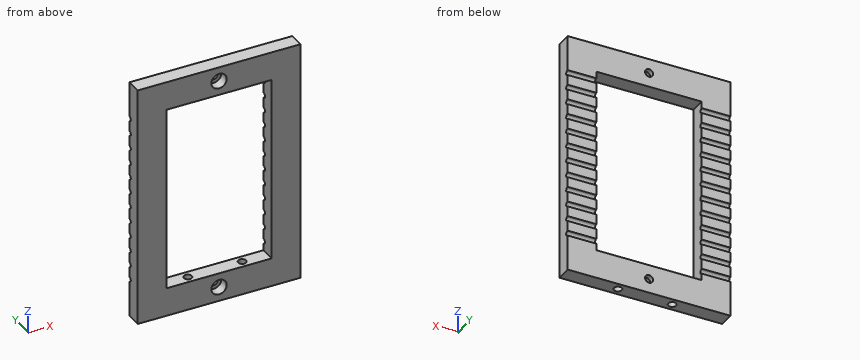
Autodesk Inventor part; units mm, degrees
ref_plane "YZ Plane" through (0, 0, 0) normal (1, 0, 0) x (0, 1, 0)
ref_plane "XZ Plane" through (0, 0, 0) normal (0, 1, 0) x (-1, 0, 0)
ref_plane "XY Plane" through (0, 0, 0) normal (0, 0, 1) x (1, 0, 0)
sketch "Sketch1" plane through (0, 0, 0) normal (0, 1, 0) x (-1, 0, 0)
  line L0 (0, 0) -> (101.6, 0)
  line L1 (101.6, 0) -> (101.6, -152.4)
  line L2 (101.6, -152.4) -> (0, -152.4)
  line L3 (0, -152.4) -> (0, 0)
  dimension "d0" = 101.6
  dimension "d1" = 152.4
extrude "Extrusion1" add sketch "Sketch1" along normal blind 9.525
sketch "Sketch2" plane through (0, 9.525, 0) normal (0, 1, 0) x (1, 0, 0)
  line L0 (-101.6, 0) -> (0, 0)
  line L1 (0, 0) -> (-17.9605, 17.9605)
  line L2 (0, 0) -> (25.4, 0) construction
  line L3 (-101.6, 152.4) -> (-101.6, 0)
  line L4 (-101.6, 152.4) -> (-83.6395, 134.4395)
  line L5 (-17.9605, 17.9605) -> (-83.6395, 17.9605)
  line L6 (-83.6395, 17.9605) -> (-83.6395, 134.4395)
  line L7 (-83.6395, 134.4395) -> (-17.9605, 134.4395)
  line L8 (-17.9605, 134.4395) -> (-17.9605, 17.9605)
  dimension "d4" = 25.4
  dimension "d5" = 135
  dimension "d6" = 25.4
extrude "Extrusion2" cut sketch "Sketch2" against normal blind 9.525 contours L5 L6 L7 L8
sketch "Sketch3" plane through (0, 0, 0) normal (1, 0, 0) x (0, 0, -1)
  line L0 (0, 9.525) -> (152.4, 9.525)
  line L1 (0, 10.079) -> (25.4, 10.079) construction
  line L2 (0, 0) -> (0, 9.525)
  line L3 (0, 9.525) -> (23.8125, 9.525)
  line L4 (134.4395, 9.525) -> (17.9605, 9.525)
  circle A0 centre (23.8125, 9.525) radius 1.5875
  circle A1 centre (33.3375, 9.525) radius 1.5875
  circle A2 centre (42.8625, 9.525) radius 1.5875
  circle A3 centre (52.3875, 9.525) radius 1.5875
  circle A4 centre (61.9125, 9.525) radius 1.5875
  circle A5 centre (71.4375, 9.525) radius 1.5875
  circle A6 centre (80.9625, 9.525) radius 1.5875
  circle A7 centre (90.4875, 9.525) radius 1.5875
  circle A8 centre (100.0125, 9.525) radius 1.5875
  circle A9 centre (109.5375, 9.525) radius 1.5875
  circle A10 centre (119.0625, 9.525) radius 1.5875
  circle A11 centre (128.5875, 9.525) radius 1.5875
  point P0 (130.175, 9.525)
  point P1 (127, 9.525)
  point P2 (120.65, 9.525)
  point P3 (117.475, 9.525)
  point P4 (101.6, 9.525)
  point P5 (98.425, 9.525)
  point P6 (82.55, 9.525)
  point P7 (79.375, 9.525)
  point P8 (73.025, 9.525)
  point P9 (69.85, 9.525)
  point P10 (63.5, 9.525)
  point P11 (60.325, 9.525)
  point P12 (53.975, 9.525)
  point P13 (50.8, 9.525)
  point P14 (44.45, 9.525)
  point P15 (41.275, 9.525)
  point P16 (34.925, 9.525)
  point P17 (31.75, 9.525)
  point P18 (22.225, 9.525)
  point P19 (25.4, 9.525)
  dimension "d11" = 23.8125
  dimension "d12" = 3.175
  dimension "d15" = 9.525
extrude "Extrusion3" cut sketch "Sketch3" against normal blind 107.95 contours L0 A0 | L0 A11 | L0 A10 | A9 L0 | L0 A9 | L0 A8 | A7 L0 | L0 A7 | L0 A6 | L0 A5 | L0 A4 | L0 A3 | L0 A2 | L0 A1 picked at (24.8555, 9.3984) picked at (128.9035, 8.9629) picked at (119.4808, 8.612) picked at (100.4308, 8.612) picked at (81.3808, 8.612) picked at (71.8558, 8.612) picked at (61.501, 9.0475) picked at (52.5145, 8.7843) picked at (42.9895, 8.7843) picked at (33.5251, 8.5384)
sketch "Sketch4" plane through (0, 0, -152.4) normal (0, 0, -1) x (-1, 0, 0)
  line L0 (101.6, 0) -> (101.6, 9.525)
  line L1 (101.6, 4.7625) -> (67.7418, 4.7625)
  line L2 (0, 4.7625) -> (33.8582, 4.7625)
  line L3 (0, 4.7625) -> (33.8582, 4.7625) construction
  point P0 (0, 0)
  dimension "d22" = 33.8582
  dimension "d23" = 33.8582
  dimension "d24" = 0
hole "Hole1" at (-67.7418, 4.7625, -152.4) direction (0, 0, 1) diameter 4.9784 depth 25.4
hole "Hole2" at (-33.8582, 4.7625, -152.4) direction (0, 0, 1) diameter 4.9784 depth 25.4
sketch "Sketch7" plane through (0, 0, 0) normal (0, -1, 0) x (1, 0, 0)
  line L0 (-101.6, 0) -> (0, 0)
  line L1 (-50.8, 0) -> (-50.8, -17.9605)
  line L2 (-83.6395, -17.9605) -> (-17.9605, -17.9605)
  line L3 (-50.8, -17.9605) -> (-50.8, -8.9803)
  line L4 (-83.6395, -134.4395) -> (-17.9605, -134.4395)
  line L5 (-50.8, -134.4395) -> (-50.8, -152.4)
  line L6 (0, -152.4) -> (-101.6, -152.4)
  line L7 (-50.8, -152.4) -> (-50.8, -143.4197)
hole "Hole5" at (-50.8, 0, -8.9803) direction (0, 1, 0) diameter 4.9784 depth 25.4 counterbore diameter 9.525 counterbore depth 6.35
hole "Hole6" at (-50.8, 0, -143.4197) direction (0, 1, 0) diameter 4.9784 depth 25.4 counterbore diameter 9.525 counterbore depth 6.35
properties part number "side-B"
Geometry check sheet. Reference: the model listing, model coordinates, mm. Coordinates: 2 decimals unless noted, no trailing zeros. Loops run counter-clockwise (first coordinate to the right, second up) from the corner with the lowest first, then second, coordinate; pieces in that order, holes last.
Item 1: Sectioned sample at B-B, the plane z = -105.5. Record the boundary of the cut face in (x, y) (1 decimal).
Item 2: Sectioned sample at A-A, the plane x = -50.8. Count the separate pieces of the cut face and the enclosed holes in it, then the cut area to 3 significant figures.
Item 3: Thickness scan on line 1 (Z direction, x = -50.8, y = 2); line 2 (Z direction, x = -50.8, y = 8.5); line 3 (X direction, y = 4.5, z = -73.5). Record the ranges inside material, lowest first.
Item 4: Go/stop test with a flat-tipped pin: pin 1 Ø7.5 at (x, z) = (-50.8, -8.98) entering from -Y. Record where the tip stops, or that it passes through.
Check result:
1. outline: (-101.6, 0) - (-83.6, 0) - (-83.6, 9.5) - (-101.6, 9.5) - close; (-18, 0) - (0, 0) - (0, 9.5) - (-18, 9.5) - close
2. separate pieces: 4
2. enclosed holes: 0
2. area: 190 mm2
3. line 1: z = -152.4 to -148.18, -138.66 to -134.44, -17.96 to -13.74, -4.22 to 0
3. line 2: z = -152.4 to -145.91, -140.93 to -134.44, -17.96 to -11.47, -6.49 to 0
3. line 3: x = -101.6 to -83.64, -17.96 to 0
4. pin 1: stops at y = 6.35
